Answer from the drawing. Dimensions are ordinates in mm from the lowest x, y and z of the part. A direction names the side the tool comes from. Round coordinates to 2 decimals unless told otherwise and drop trailing zeros. Write each loop counter-clockwise with the first axis right and the second up, starting at its lowest first coordinate (ties: lowest second). Pieces come first, ordered by that corner, then holes. Notation, with made-up numbers: (-34, 12.5) - (2, 12.5) arc R11 ccw to (2, 32.5) - close; hole circle Ø3 at (-33.75, 0.5). An arc over 180 degrees is marked (long way). Answer as CSV lines item,"result". Start each with the question number.
1) Consider line 1 along Y through (x, z) = (15, 2.7) (1 decimal); line 2 along X through (y, z) = (90.5, 7.5); line 3 along X through (y, z) = (5, 8.75). Determine where each line is inside the solid, lowest interval first.
2) For a pull along X with two mould halves and no side action, classify the marked faces 1, 2, 3 and 4 as +X half, -X half, draft (parallel to the pull), parting line (faces both ways), or undercut.
3) Find section A-A on x = 22.5. Determine the outline of the cut face in (y, z), then the cut area to 3 significant figures.
4) Each of these flat-tipped pins is pushed along its axis until it touches: pin 1 (3 mm diameter, centred on x = 15, y = 80.28, fed in from -Z); pin 2 (7.5 mm diameter, centred on x = 17.5, z = 16, fed in from -Y); pin 3 (3 mm diameter, centred on x = 16, y = 18.5, fed in from +Z). Where does it stop, or does it pass through?
5) Find section D-D on x = 15. Determine the outline of the cut face in (y, z) (1 decimal), then the cut area to 3 significant figures.
6) Find section B-B on z = 11.75. Determine the outline of the cut face in (x, y), then the cut area to 3 significant figures.
7) Find section C-C on y = 44.5. Determine the outline of the cut face in (x, z), then the cut area to 3 significant figures.
8) Which of the six approach directions +Z, -Z, +X, -X, +Y, -Y give full straight-line access (tool end or side, diameter ignored) to the marked faces 5, 6, 7 and 8?
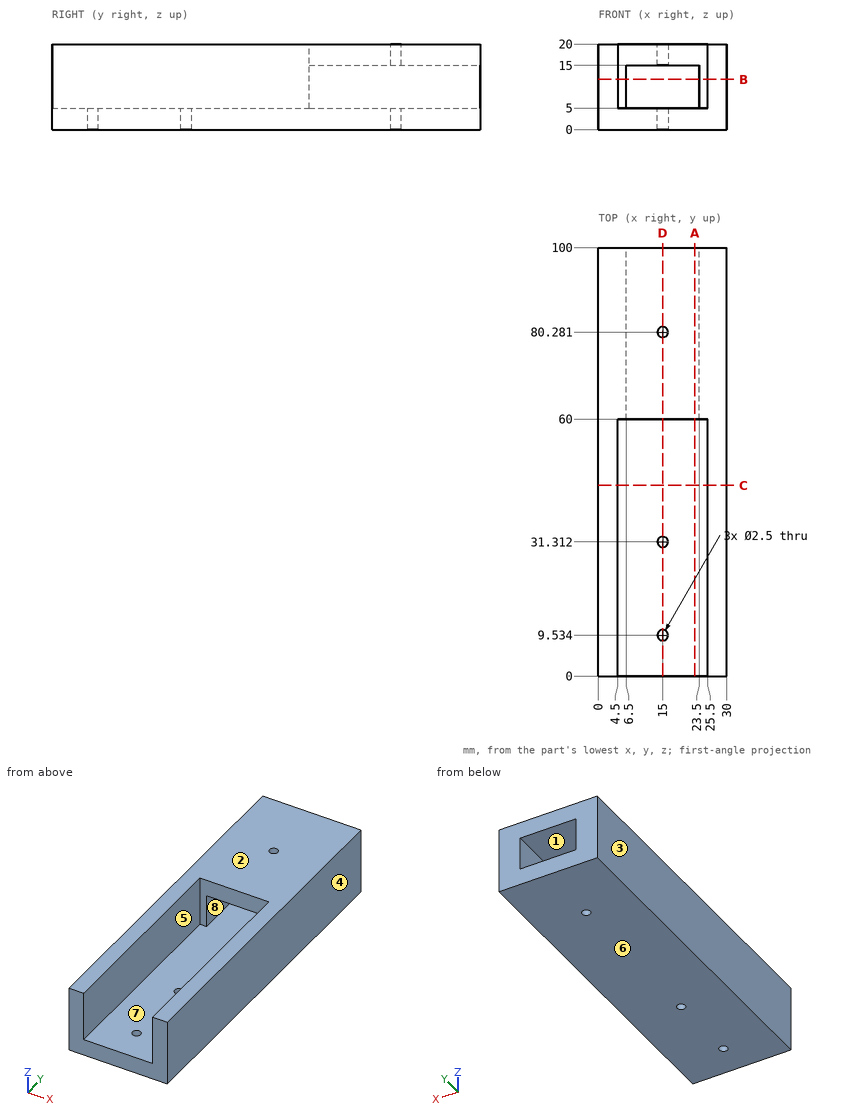
Check values:
1,line 1,"y = 0 to 8.3, 10.8 to 30.1, 32.6 to 79, 81.5 to 100"
1,line 2,"x = 0 to 6.5, 23.5 to 30"
1,line 3,"x = 0 to 4.5, 25.5 to 30"
2,face 1,"undercut"
2,face 2,"draft"
2,face 3,"-X half"
2,face 4,"+X half"
3,outline,"(0, 0) - (100, 0) - (100, 5) - (0, 5) - close; (60, 15) - (100, 15) - (100, 20) - (60, 20) - close"
3,area,"700 mm^2"
4,pin 1,"stops at z = 0"
4,pin 2,"stops at y = 60"
4,pin 3,"stops at z = 5"
5,outline,"(0, 0) - (8.3, 0) - (8.3, 5) - (0, 5) - close; (10.8, 0) - (30.1, 0) - (30.1, 5) - (10.8, 5) - close; (32.6, 0) - (79, 0) - (79, 5) - (32.6, 5) - close; (60, 15) - (79, 15) - (79, 20) - (60, 20) - close; (81.5, 0) - (100, 0) - (100, 5) - (81.5, 5) - close; (81.5, 15) - (100, 15) - (100, 20) - (81.5, 20) - close"
5,area,"650 mm^2"
6,outline,"(0, 0) - (4.5, 0) - (4.5, 60) - (6.5, 60) - (6.5, 100) - (0, 100) - close; (23.5, 60) - (25.5, 60) - (25.5, 0) - (30, 0) - (30, 100) - (23.5, 100) - close"
6,area,"1,060 mm^2"
7,outline,"(0, 0) - (30, 0) - (30, 20) - (25.5, 20) - (25.5, 5) - (4.5, 5) - (4.5, 20) - (0, 20) - close"
7,area,"285 mm^2"
8,face 5,"+Z, -Y"
8,face 6,"-Z, +X, -X, +Y, -Y"
8,face 7,"-Y"
8,face 8,"+Y, -Y"
